Read the model definition and answer for the solid it produces. Units are mm, in the model's axes. Face numbers are marked on the shaded views. A direction names the side the tool comes from. Give positions to 0.01 mm unless a question says otherwise; leave off trailing zeros. Loops run counter-clockwise (first coordinate to the right, second up) from the corner with the lowest first, then second, coordinate; pieces in that order, holes last.
(1) Find section D-D, the plane z = -11.5. Write down the section's boundary in (x, y).
(2) Each of these flat-tipped pins is pushed along its axis until it touches: P1, Ø7.5, axis at y = 9.5, z = -7.5, coming from the +X side; P2, Ø8, axis at x = -26, z = 7.5, coming from the +Y side; P3, Ø4.5, axis at x = -8.5, y = 7, coming from the -Z side; P4, Ø2.5, axis at x = 13.91, z = -12.15, coming from the -Y side. Where does it stop, or does it pass through?
(3) Find section C-C, the plane z = 17. Write down the section's boundary in (x, y).
(4) Find section B-B, the plane x = -5. Write down the section's boundary in (y, z), then the cut area to 3 significant figures.
(5) Find section A-A, the plane y = 2.75. Write down the section's boundary in (x, z).
(6) Which of the six approach directions +Z, -Z, +X, -X, +Y, -Y give full straight-line access (tool end or side, diameter ignored) to the marked faces 1, 2, 3, 4 and 5?
(7) Straight lines are drawn through the part: probe 1 along Z at (x, y) = (-12.5, 15.75); probe 2 along Y at (x, z) = (-11.5, 21); probe 3 along X at (y, z) = (3.75, 18.5). For each, find the intervals that lie inside material, in ascending order.
```python
from build123d import *

# Parameters (mm, degrees)
SKETCH1_W           = 50.6
SKETCH1_H           = 38.52
SKETCH1_R           = 1.5
BOSS_EXTRUDE1_DEPTH = 1.6
FILLET1_R           = 3
FILLET2_R           = 3
FILLET3_R           = 3
FILLET4_R           = 3
SKETCH2_W           = 18.8
SKETCH2_H           = 15
BOSS_EXTRUDE2_DEPTH = 15.5


with BuildPart() as part:
    # Sketch1 → Boss-Extrude1 (new body)
    with BuildSketch(Plane(origin=(0, 0, 0), x_dir=(1, 0, 0), z_dir=(0, 1, 0))):
        with Locations((-8.389974293, -4.106015424)):
            Rectangle(SKETCH1_W, SKETCH1_H)
        with Locations(Location((13.910025707, 12.153984576, 0), (0, 0, 270))):
            Circle(SKETCH1_R, mode=Mode.SUBTRACT)
        with Locations(Location((13.910025707, -20.366015424, 0), (0, 0, 270))):
            Circle(SKETCH1_R, mode=Mode.SUBTRACT)
        with Locations(Location((-30.689974293, -20.366015424, 0), (0, 0, 270))):
            Circle(SKETCH1_R, mode=Mode.SUBTRACT)
        with Locations(Location((-30.689974293, 12.153984576, 0), (0, 0, 270))):
            Circle(SKETCH1_R, mode=Mode.SUBTRACT)
    extrude(amount=BOSS_EXTRUDE1_DEPTH)

    # Fillet1
    fillet1_edges = [part.edges().sort_by_distance(p)[0] for p in [
        (16.910025707, 0.8, -15.153984576),
    ]]
    fillet(fillet1_edges, radius=FILLET1_R)

    # Fillet2
    fillet2_edges = [part.edges().sort_by_distance(p)[0] for p in [
        (-33.689974293, 0.8, -15.153984576),
    ]]
    fillet(fillet2_edges, radius=FILLET2_R)

    # Fillet3
    fillet3_edges = [part.edges().sort_by_distance(p)[0] for p in [
        (-33.689974293, 0.8, 23.366015424),
    ]]
    fillet(fillet3_edges, radius=FILLET3_R)

    # Fillet4
    fillet4_edges = [part.edges().sort_by_distance(p)[0] for p in [
        (16.910025707, 0.8, 23.366015424),
    ]]
    fillet(fillet4_edges, radius=FILLET4_R)

    # Sketch2 → Boss-Extrude2 (add)
    with BuildSketch(Plane(origin=(0, 1.6, 0), x_dir=(1, 0, 0), z_dir=(0, 1, 0))):
        with Locations((-11.789974293, 4.653984576)):
            Rectangle(SKETCH2_W, SKETCH2_H)
        with Locations((-11.789974293, -12.866015424)):
            Rectangle(SKETCH2_W, SKETCH2_H)
    extrude(amount=BOSS_EXTRUDE2_DEPTH)


solid = part.part
```
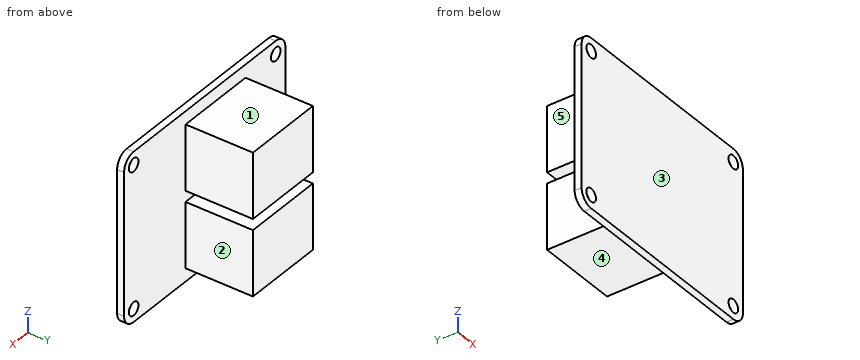
Entries:
1. outline: (-33.69, 0) - (-32.04, 0) - (-32.04, 1.6) - (-33.69, 1.6) - close; (-29.34, 0) - (12.56, 0) - (12.56, 1.6) - (-2.39, 1.6) - (-2.39, 17.1) - (-21.19, 17.1) - (-21.19, 1.6) - (-29.34, 1.6) - close; (15.26, 0) - (16.91, 0) - (16.91, 1.6) - (15.26, 1.6) - close
2. P1: stops at x = -2.39
2. P2: stops at y = 1.6
2. P3: stops at z = -12.15
2. P4: passes through
3. outline: (-33.69, 0) - (16.91, 0) - (16.91, 1.6) - (-2.39, 1.6) - (-2.39, 17.1) - (-21.19, 17.1) - (-21.19, 1.6) - (-33.69, 1.6) - close
4. outline: (0, -15.15) - (1.6, -15.15) - (1.6, -12.15) - (17.1, -12.15) - (17.1, 2.85) - (1.6, 2.85) - (1.6, 5.37) - (17.1, 5.37) - (17.1, 20.37) - (1.6, 20.37) - (1.6, 23.37) - (0, 23.37) - close
4. area: 527 mm2
5. outline: (-21.19, -12.15) - (-2.39, -12.15) - (-2.39, 2.85) - (-21.19, 2.85) - close; (-21.19, 5.37) - (-2.39, 5.37) - (-2.39, 20.37) - (-21.19, 20.37) - close
6. face 1: +Z, +X, -X, +Y
6. face 2: +Z, -Z, +X, +Y
6. face 3: +Z, -Z, +X, -X, -Y
6. face 4: -Z, +X, -X, +Y
6. face 5: +Z, -Z, -X, +Y
7. probe 1: z = -12.15 to 2.85, 5.37 to 20.37
7. probe 2: y = 0 to 1.6
7. probe 3: x = -21.19 to -2.39
